Autodesk Inventor part; units mm, degrees
ref_plane "YZ Plane" through (0, 0, 0) normal (1, 0, 0) x (0, 1, 0)
ref_plane "XZ Plane" through (0, 0, 0) normal (0, 1, 0) x (-1, 0, 0)
ref_plane "XY Plane" through (0, 0, 0) normal (0, 0, 1) x (1, 0, 0)
sketch "Sketch1" plane through (0, 0, 0) normal (0, 0, 1) x (1, 0, 0)
  circle A0 centre (0, 0) radius 2.5
  circle A1 centre (0, 0) radius 1.9202
  point P0 (0, 0)
extrude "Extrusion1" add sketch "Sketch1" against normal blind 5
sketch "Sketch2" plane through (0, 0, 0) normal (0, 0, 1) x (1, 0, 0)
  circle A0 centre (0, 0) radius 1.9202
  circle A1 centre (0, 0) radius 2.5
  point P0 (0, 0)
extrude "Extrusion2" add sketch "Sketch2" along normal blind 1
sketch "Sketch3" plane through (0, 0, 1) normal (0, 0, 1) x (1, 0, 0)
  circle A0 centre (0, 0) radius 1.9202
  circle A1 centre (0, 0) radius 2.5
  ellipse E0 centre (0, 0) end of major axis (-5.3322, 0) minor radius 4.4331
  point P0 (0, 0)
extrude "Extrusion3" add sketch "Sketch3" along normal blind 1 contours A1 | E0
sketch "Sketch4" plane through (0, 0, 2) normal (0, 0, 1) x (1, 0, 0)
  circle A0 centre (0, 0) radius 2.322
extrude "Extrusion4" cut sketch "Sketch4" against normal through all
properties part number "Pushfit-adapter-cap"
The model under review builds one solid part; all positions refer to its coordinate system, in mm. Round coordinates to 2 decimals unless told otherwise and drop trailing zeros. Loops run counter-clockwise (first coordinate to the right, second up) from the corner with the lowest first, then second, coordinate; pieces in that order, holes last. Notation, with made-up numbers: (43.5, 12) - (75.5, 12) arc R31 ccw to (75.5, 38) - close; hole circle Ø3 at (62.5, -2.5). An arc over 180 degrees is marked (long way). Use a Markdown table: item, result. Add a question column.
Q1. Insertion check: pin 1 Ø4 at (x, y) = (0, 0) entering from -Z. The pin has a flat end and moves straight along its axis. Give the tip position at first contact, or say it passes through.
Q2. Add section A-A (z = -2.25). State the section outline as (x, y) points.
Q3. For probe 1 along Y at (x, z) = (0, -1.25); probe 2 along Z at (x, y) = (2.5, -2); probe 3 along Y at (x, z) = (1, -4.25), list the stretches that pass through material, from the lowest coordinate up.
Q4. The part is to be moulded in two halves that separate along X. For faces 1 (the face through (-2.44, 1.05, 1)), 2 (the face through (-0.54, -2.44, -1.96)), 3 (the face through (2.215, 0.697, -1.451)), say which applies: pulls with the +X half, pulls with the -X half, needs draft (parallel to the pull), parting line crosses it, or undercut.
Worked answers:
| question | item | result |
|---|---|---|
| 1 | pin 1 | through |
| 2 | outline | circle Ø5 at (0, 0); hole circle Ø4.64 at (0, 0) |
| 3 | probe 1 | -2.5 to -2.32, 2.32 to 2.5 |
| 3 | probe 2 | 1 to 2 |
| 3 | probe 3 | -2.29 to -2.1, 2.1 to 2.29 |
| 4 | face 1 | needs draft |
| 4 | face 2 | parting line crosses it |
| 4 | face 3 | undercut |
